```python
from build123d import *

# Parameters (mm, degrees)
RESSALTO_EXTRUS_O1_DEPTH = 15
ESBO_O2_R                = 1.8
CORTE_EXTRUS_O1_DEPTH    = 33.592176975
ESBO_O3_W                = 9.75
ESBO_O3_H                = 3
CORTE_EXTRUS_O2_DEPTH    = 3
FILETE1_R                = 0.2
CHANFRO1_SIZE            = 1


with BuildPart() as part:
    # Esboço1 → Ressalto-extrusão1 (new, symmetric)
    with BuildSketch(Plane.XY):
        with BuildLine():
            Line((-22.5, 0), (22.5, 0))
            Line((22.5, 0), (28.5, 0))
            Line((28.5, 0), (28.5, 5))
            Line((28.5, 5), (22.5, 5))
            ThreePointArc((22.5, 5), (18.75, 1.25), (15, 5))
            ThreePointArc((15, 5), (11.25, 1.25), (7.5, 5))
            ThreePointArc((7.5, 5), (3.75, 1.25), (0, 5))
            ThreePointArc((0, 5), (-3.75, 1.25), (-7.5, 5))
            ThreePointArc((-7.5, 5), (-11.25, 1.25), (-15, 5))
            ThreePointArc((-15, 5), (-18.75, 1.25), (-22.5, 5))
            Line((-22.5, 5), (-28.5, 5))
            Line((-28.5, 5), (-28.5, 0))
            Line((-28.5, 0), (-22.5, 0))
        make_face()
    extrude(amount=RESSALTO_EXTRUS_O1_DEPTH, both=True)

    # Esboço2 → Corte-extrusão1 (cut, through all)
    with BuildSketch(Plane(origin=(0, 5, 0), x_dir=(1, 0, 0), z_dir=(0, 1, 0))):
        with Locations(Location((-25.5, 0, 0), (0, 0, 180))):
            Circle(ESBO_O2_R)
        with Locations((25.5, 0)):
            Circle(ESBO_O2_R)
    extrude(amount=-CORTE_EXTRUS_O1_DEPTH, mode=Mode.SUBTRACT)

    # Esboço3 → Corte-extrusão2 (cut)
    with BuildSketch(Plane(origin=(0, 5, 0), x_dir=(1, 0, 0), z_dir=(0, 1, 0))):
        with Locations((-23.625, 13.5)):
            Rectangle(ESBO_O3_W, ESBO_O3_H)
        with Locations((-23.625, -13.5)):
            Rectangle(ESBO_O3_W, ESBO_O3_H)
        with Locations((23.625, -13.5)):
            Rectangle(ESBO_O3_W, ESBO_O3_H)
        with Locations((23.625, 13.5)):
            Rectangle(ESBO_O3_W, ESBO_O3_H)
    extrude(amount=-CORTE_EXTRUS_O2_DEPTH, mode=Mode.SUBTRACT)

    # Filete1
    filete1_edges = [part.edges().sort_by_distance(p)[0] for p in [
        (-15, 5, 0),
        (-7.5, 5, 0),
        (0, 5, 0),
        (7.5, 5, 0),
        (15, 5, 0),
    ]]
    fillet(filete1_edges, radius=FILETE1_R)

    # Chanfro1
    chanfro1_edges = [part.edges().sort_by_distance(p)[0] for p in [
        (-23.7, 0, 0),
        (23.7, 0, 0),
        (23.7, 5, 0),
    ]]
    chamfer(chanfro1_edges, length=CHANFRO1_SIZE)


solid = part.part
```
Here's how the part is built. I have some questions about the finished solid (model axes, mm). A direction names the side the tool comes from. Give positions to 0.01 mm unless a question says otherwise; leave off trailing zeros. Loops run counter-clockwise (first coordinate to the right, second up) from the corner with the lowest first, then second, coordinate; pieces in that order, holes last. Notation, with made-up numbers: M 23,76 L 36,76 A30 cw 36,100 Z; hole C 41,35 d2. An arc over 180 degrees is marked long. Use one line per item in the form item = value. Start each with the question number.
Q1. Will these pins go through, and if not, where does the flat tip stop? pin 1 Ø0.9 at (x, y) = (24.5, 4) entering from +Z; pin 2 Ø1.5 at (x, y) = (24, 4) entering from -Z; pin 3 Ø12 at (x, z) = (7, -3.5) entering from +Y.
Q2. If we section it at C-C (x = 25.5): Write out the boundary of the cut face in (y, z).
Q3. If we section it at A-A (x = -25.5): Write out the boundary of the cut face in (y, z), then the cut area to 3 significant figures.
Q4. Thinking about a two-plate mould opening in Z: for faces 1 (the cylindrical face through (27.217, 2.521, -0.541)), 2 (the flat face through (28.5, 2, 0)), 3 (the flat face through (26, 4, -12)), which applies, +Z half, -Z half, draft (parallel to the pull), parting line (faces both ways), or undercut?
Q5. If we section it at B-B (y = 2.7): State how many separate pieces and enclosed holes the cut face has, then the cut area to 3 significant figures.
Q6. Which directions (+Z, -Z, +X, -X, +Y, -Y) give clear straight access to the entire face, cutting with the end or side of a thin tool? Please do faces 4 (the flat face through (26, 4, 12)), 5 (the flat face through (25, 2, -14)), 6 (the flat face through (-26, 4, -12)), 7 (the flat face through (-26, 4, 12)).
Q7. I need wall thicknesses on line 1 along Z through (x, y) = (-25.5, 3.45); line 2 along Y through (x, z) = (-19, 8.5); line 3 along Z through (x, y) = (25, 1.45). Which ranges of each line are inside material? Lowest first, please.
Taken from the geometry:
q1.pin_1 = 12
q1.pin_2 = -12
q1.pin_3 = 3.96
q2.outline = M 0,-15 L 2,-15 L 2,-12 L 5,-12 L 5,-2.8 L 4,-1.8 L 1,-1.8 L 0,-2.8 Z; M 0,2.8 L 1,1.8 L 4,1.8 L 5,2.8 L 5,12 L 2,12 L 2,15 L 0,15 Z
q3.outline = M 0,-15 L 2,-15 L 2,-12 L 5,-12 L 5,-1.8 L 1,-1.8 L 0,-2.8 Z; M 0,2.8 L 1,1.8 L 5,1.8 L 5,12 L 2,12 L 2,15 L 0,15 Z
q3.area = 113 mm^2
q4.face_1 = undercut
q4.face_2 = draft
q4.face_3 = -Z half
q5.separate_pieces = 7
q5.enclosed_holes = 2
q5.area = 542 mm^2
q6.face_4 = +Z, +X, +Y
q6.face_5 = -Z, +X, +Y
q6.face_6 = -Z, -X, +Y
q6.face_7 = +Z, -X, +Y
q7.line_1 = -12 to -1.8, 1.8 to 12
q7.line_2 = 0 to 1.26
q7.line_3 = -15 to -1.73, 1.73 to 15
